Check sheet for the modelled part. Datum: model origin and axes. Units: mm. A direction names the side the tool comes from. Round coordinates to 2 decimals unless told otherwise and drop trailing zeros. Loops run counter-clockwise (first coordinate to the right, second up) from the corner with the lowest first, then second, coordinate; pieces in that order, holes last. Notation, with made-up numbers: (9, -3.75) - (25, -3.75) arc R22 ccw to (25, 19.25) - close; hole circle Ø11 at (-22.5, 89.5). An arc over 180 degrees is marked (long way). Return JSON: item names as keys, results as strings.
from build123d import *

# Parameters (mm, degrees)
SKETCH_1_W          = 21
SKETCH_1_H          = 24
EXTRUDE_1_DEPTH     = 1.5
SKETCH_2_R          = 1.75
CUT_EXTRUDE_1_DEPTH = 1.5
SKETCH_3_R          = 2.5
EXTRUDE_2_DEPTH     = 5


with BuildPart() as part:
    # 草图1 → 凸台-拉伸1 (new body)
    with BuildSketch(Plane(origin=(0, 0, 0), x_dir=(1, 0, 0), z_dir=(0, 1, 0))):
        Rectangle(SKETCH_1_W, SKETCH_1_H)
    extrude(amount=EXTRUDE_1_DEPTH)

    # 草图2 → 切除-拉伸1 (cut)
    with BuildSketch(Plane(origin=(0, 1.5, 0), x_dir=(1, 0, 0), z_dir=(0, 1, 0))):
        with Locations(Location((-7.5, 8.800641953, 0), (0, 0, 270))):
            Circle(SKETCH_2_R)
        with Locations(Location((7.5, 8.800641953, 0), (0, 0, 270))):
            Circle(SKETCH_2_R)
    extrude(amount=-CUT_EXTRUDE_1_DEPTH, mode=Mode.SUBTRACT)

    # 草图3 → 凸台-拉伸2 (add)
    with BuildSketch(Plane(origin=(0, 1.5, 0), x_dir=(1, 0, 0), z_dir=(0, 1, 0))):
        with Locations(Location((-4.607665944, -5.298815836, 0), (0, 0, 270))):
            Circle(SKETCH_3_R)
        with Locations(Location((4.607665944, -5.298815836, 0), (0, 0, 270))):
            Circle(SKETCH_3_R)
    extrude(amount=EXTRUDE_2_DEPTH)


solid = part.part
Q1. Depth check by flat-ended pin: P1, Ø1, axis at x = 5.5, y = 2.5, coming from the +Z side; P2, Ø10.5, axis at x = 1, z = 2, coming from the +Y side; P3, Ø4.5, axis at x = -7.5, z = -8.8, coming from the +Y side. Enter the tip coordinate at first touch or a pass-through.
Answer key:
{"P1": "stops at z = 7.77", "P2": "stops at y = 6.5", "P3": "stops at y = 1.5"}
Q2. Sectioned sample at B-B (z = -9.5). Enter the section's corners in (x, y), plus the area to 3 significant figures.
Answer key:
{"outline": "(-10.5, 0) - (-9.1, 0) - (-9.1, 1.5) - (-10.5, 1.5) - close; (-5.9, 0) - (5.9, 0) - (5.9, 1.5) - (-5.9, 1.5) - close; (9.1, 0) - (10.5, 0) - (10.5, 1.5) - (9.1, 1.5) - close", "area": "21.9 mm²"}
Q3. Sectioned sample at C-C (x = 5). Enter the section's corners in (y, z), plus the area to 3 significant figures.
Answer key:
{"outline": "(0, -12) - (1.5, -12) - (1.5, 2.83) - (6.5, 2.83) - (6.5, 7.77) - (1.5, 7.77) - (1.5, 12) - (0, 12) - close", "area": "60.7 mm²"}
Q4. Tool access check on faces 5 (the face through (-4.5, 4, 2.8)), 6 (the face through (10.5, 1, 0)). Record the directions out of +Z, -Z, +X, -X, +Y, -Y that give a thin tool (end or side, any length) a straight path to the whole face; none if there is none.
Answer key:
{"face 5": "+Y", "face 6": "+Z, -Z, +X, +Y, -Y"}
Q5. Sectioned sample at A-A (x = -7.5). Enter the section's corners in (y, z).
Answer key:
{"outline": "(0, -12) - (1.5, -12) - (1.5, -10.55) - (0, -10.55) - close; (0, -7.05) - (1.5, -7.05) - (1.5, 12) - (0, 12) - close"}
Q6. Scan lines: probe 1 along Y at (x, z) = (-2, -11); probe 2 along Z at (x, y) = (-4.5, 3.75); probe 3 along Z at (x, y) = (2.75, 5.75). Record each from-to range of solid material in increasing order. Write a range as [from, to].
Answer key:
{"probe 1": "y = [0, 1.5]", "probe 2": "z = [2.8, 7.8]", "probe 3": "z = [3.63, 6.97]"}
Q7. Sectioned sample at D-D (y = 6). Enter the section's corners in (x, z), plus the area to 3 significant figures.
Answer key:
{"outline": "circle Ø5 at (-4.61, 5.3); circle Ø5 at (4.61, 5.3)", "area": "39.3 mm²"}
Q8. Draft check along X on faces 1 (the face through (0, 1, -12)), 2 (the face through (6.3, 3.96, 3.46)), 3 (the face through (-10.5, 1, 0)), 4 (the face through (6.83, 0.76, -7.184)). Enter one of: released by +X, released by -X, zero draft, split by the parting line, or undercut.
Answer key:
{"face 1": "zero draft", "face 2": "undercut", "face 3": "released by -X", "face 4": "undercut"}
